Source: CAD feature listing. Evaluate the final solid. Frame: model axes, mm. A direction names the side the tool comes from. Round coordinates to 2 decimals unless told otherwise and drop trailing zeros. Write each loop counter-clockwise with the first axis right and the second up, starting at its lowest first coordinate (ties: lowest second). Pieces come first, ordered by that corner, then holes. Notation, with made-up numbers: (-32.5, 78) -> (5.5, 78) arc R25 cw to (5.5, 102) -> close; hole circle Ø1 at (13.25, -31). An arc over 180 degrees is marked (long way). Put each result on its own line as item: value.
```python
from build123d import *

# Parameters (mm, degrees)
F0_W     = 254
F0_H     = 254
F1_DEPTH = 254
F4_T     = -50.8
F5_R     = 69.85
F6_DEPTH = 254.001
F7_W     = 50.8
F7_H     = 50.8
F8_DEPTH = 114.3


with BuildPart() as f1:
    # F0 (on Top) → F1 (new body)
    with BuildSketch(Plane.XY):
        with Locations((127, -127)):
            Rectangle(F0_W, F0_H)
    extrude(amount=F1_DEPTH)

    # F4
    f4_openings = [f1.faces().sort_by_distance(p)[0] for p in [
        (127, -254, 127),
        (254, -127, 127),
        (127, -127, 254),
    ]]
    offset(amount=F4_T, openings=f4_openings)

    # F5 (on Front) → F6 (cut, through all)
    with BuildSketch(Plane.XZ):
        with Locations((152.4, 152.4)):
            Circle(F5_R)
    extrude(amount=F6_DEPTH, mode=Mode.SUBTRACT)

    # F7 (on Top) → F8 (join)
    with BuildSketch(Plane.XY):
        with Locations((127, -165.1)):
            Rectangle(F7_W, F7_H)
    extrude(amount=F8_DEPTH)


solid = f1.part
```
Q1. Reachability of faces 4 (the flat face through (69, -254, 41)), 5 (the flat face through (152.4, -165, 82)), 6 (the flat face through (127, -139.7, 82)) from +Z, -Z, +X, -X, +Y, -Y: full face, straight path, thin tool, end or side. Return the list, or none.
Ans:
face 4: +Z, -Z, +X, -X, -Y
face 5: +Z, +X, -Y
face 6: +Z, +X
Q2. Material intervals for line 1 (Z direction, x = 152.4, y = -18.5); line 2 (Y direction, x = 113, z = 74); line 3 (X direction, y = -153.5, z = 91), sorted ascending. Write a range as [from, to].
Ans:
line 1: z = [0, 82.55], [222.25, 254]
line 2: y = [-190.5, -139.7], [-50.8, 0]
line 3: x = [0, 50.8], [101.6, 152.4]
Q3. Cut plane C-C on z = 235.5. Output: boundary loops of the cut face in (x, y), and give its area (3 significant figures).
Ans:
outline: (0, -254) -> (50.8, -254) -> (50.8, -50.8) -> (254, -50.8) -> (254, 0) -> (0, 0) -> close
area: 23,200 mm^2
Q4. Cut plane D-D on z = 187.5. Output: boundary loops of the cut face in (x, y), and give its area (3 significant figures).
Ans:
outline: (0, -254) -> (50.8, -254) -> (50.8, -50.8) -> (92.01, -50.8) -> (92.01, 0) -> (0, 0) -> close; (212.79, -50.8) -> (254, -50.8) -> (254, 0) -> (212.79, 0) -> close
area: 17,100 mm^2
Q5. Cut plane B-B on y = -40. Output: boundary loops of the cut face in (x, z), and give its area (3 significant figures).
Ans:
outline: (0, 0) -> (254, 0) -> (254, 254) -> (0, 254) -> close; hole circle Ø139.7 at (152.4, 152.4)
area: 49,200 mm^2
Q6. Pin query (flat end, axial travel): pin 1 (6 mm diameter, centred on x = 79.5, y = -145, fed in from +Z); pin 2 (5 mm diameter, centred on y = -78, z = 157.5, fed in from +X); pin 3 (1 mm diameter, centred on y = -170.5, z = 56.5, fed in from +X). Return the tip coordinate at first contact, or that it passes through.
Ans:
pin 1: stops at z = 50.8
pin 2: stops at x = 50.8
pin 3: stops at x = 152.4
Q7. Draft query along X for faces 1 (the flat face through (101.6, -165, 82)), 2 (the flat face through (127, -165, 114.3)), 3 (the flat face through (254, -72, 41)). Return one class per face: +X half, -X half, draft (parallel to the pull), parting line (faces both ways), or undercut.
Ans:
face 1: undercut
face 2: draft
face 3: +X half
Q8. Cut plane A-A on z = 152.4. Output: boundary loops of the cut face in (x, y), and give its area (3 significant figures).
Ans:
outline: (0, -254) -> (50.8, -254) -> (50.8, -50.8) -> (82.55, -50.8) -> (82.55, 0) -> (0, 0) -> close; (222.25, -50.8) -> (254, -50.8) -> (254, 0) -> (222.25, 0) -> close
area: 16,100 mm^2
